```python
from build123d import *

# Parameters (mm, degrees)
F0_W     = 13
F0_H     = 25
F0_W_2   = 20
F0_H_2   = 15
F1_DEPTH = 2


with BuildPart() as f1:
    # F0 (on Front) → F1 (new body)
    with BuildSketch(Plane.XZ):
        Polygon((40.276188, 34.517385), (-59.723812, 34.517385), (-59.723812, -33.482615), (-43.465011, -33.482615), (-43.465011, -10.482615), (-32.465011, -10.482615), (-32.465011, -33.482615), (40.276188, -33.482615), align=None)
        with Locations((-6.950044, -12.5)):
            Rectangle(F0_W, F0_H, mode=Mode.SUBTRACT)
        with Locations((15.719853, -12.5)):
            Rectangle(F0_W, F0_H, mode=Mode.SUBTRACT)
        with Locations((-42.465011, 18.383584)):
            Rectangle(F0_W_2, F0_H_2, mode=Mode.SUBTRACT)
        with Locations((-10.450044, 18.383584)):
            Rectangle(F0_W_2, F0_H_2, mode=Mode.SUBTRACT)
        with Locations((18.867977, 18.383584)):
            Rectangle(F0_W_2, F0_H_2, mode=Mode.SUBTRACT)
    extrude(amount=F1_DEPTH)


solid = f1.part
```
Geometry: final body of the model. Coordinates: model frame, mm. A direction names the side the tool comes from. Coordinates: 2 decimals unless noted, no trailing zeros. Order: outer loops, then holes, each group sorted by start corner. A loop starts at its lowest first (then second) coordinate and runs counter-clockwise, first axis right, second up. Notation, with made-up numbers: M 75.5,51.25 L 102.5,51.25 A9 ccw 102.5,56.25 Z; hole C -20,-1.75 d11. An arc over 180 degrees is marked long. Answer as CSV lines item,"result".
Q1. Section C-C on z = -27.5. Return the cut outline in (x, y).
Answers:
outline,"M -59.72,-2 L -43.47,-2 L -43.47,0 L -59.72,0 Z; M -32.47,-2 L 40.28,-2 L 40.28,0 L -32.47,0 Z"
Q2. Set-up query: faces 1 (the flat face through (-10, -2, 1)), 2 (the flat face through (19, -1, 10.884)), 3 (the flat face through (-38, -1, -10.483)). Return all of +Z, -Z, +X, -X, +Y, -Y with unobstructed straight access to the full face (end or side cutting, diameter ignored); none if empty.
Answers:
face 1,"+Z, -Z, +X, -X, -Y"
face 2,"+Y, -Y"
face 3,"-Z, +Y, -Y"
Q3. First-contact query: P1, Ø8, axis at x = -11.5, z = -21, coming from the -Y side; P2, Ø1, axis at x = -41.5, y = -1, coming from the -Z side. Flat tips, straight axial feed; report the tip coordinate or a pass-through.
Answers:
P1,"stops at y = -2"
P2,"stops at z = -10.48"
Q4. Section B-B on x = -38. Return the cut outline in (y, z).
Answers:
outline,"M -2,-10.48 L 0,-10.48 L 0,10.88 L -2,10.88 Z; M -2,25.88 L 0,25.88 L 0,34.52 L -2,34.52 Z"
Q5. Line query: probe 1 along X at (y, z) = (-0.75, -6.5); probe 2 along Z at (x, y) = (-1.5, -1.35); probe 3 along X at (y, z) = (-0.4, -14). Output: solid intervals per line, ascending. Write a range as [from, to].
Answers:
probe 1,"x = [-59.72, -13.45], [-0.45, 9.22], [22.22, 40.28]"
probe 2,"z = [-33.48, -25], [0, 10.88], [25.88, 34.52]"
probe 3,"x = [-59.72, -43.47], [-32.47, -13.45], [-0.45, 9.22], [22.22, 40.28]"
Q6. Section A-A on z = -2.5. Return the cut outline in (x, y).
Answers:
outline,"M -59.72,-2 L -13.45,-2 L -13.45,0 L -59.72,0 Z; M -0.45,-2 L 9.22,-2 L 9.22,0 L -0.45,0 Z; M 22.22,-2 L 40.28,-2 L 40.28,0 L 22.22,0 Z"
Q7. Draft query along Z for faces 4 (the flat face through (8.868, -1, 18)), 5 (the flat face through (-10, 0, 1)), 6 (the flat face through (3, -1, -33.483)). Return one class per face: pulls with the +Z half, pulls with the -Z half, needs draft (parallel to the pull), parting line crosses it, or undercut.
Answers:
face 4,"undercut"
face 5,"needs draft"
face 6,"pulls with the -Z half"
Q8. Section D-D on y = -1.05. Return the cut outline in (x, z), and give its area (3 significant figures).
Answers:
outline,"M -59.72,-33.48 L -43.47,-33.48 L -43.47,-10.48 L -32.47,-10.48 L -32.47,-33.48 L 40.28,-33.48 L 40.28,34.52 L -59.72,34.52 Z; hole M -52.47,10.88 L -32.47,10.88 L -32.47,25.88 L -52.47,25.88 Z; hole M -20.45,10.88 L -0.45,10.88 L -0.45,25.88 L -20.45,25.88 Z; hole M -13.45,-25 L -0.45,-25 L -0.45,0 L -13.45,0 Z; hole M 8.87,10.88 L 28.87,10.88 L 28.87,25.88 L 8.87,25.88 Z; hole M 9.22,-25 L 22.22,-25 L 22.22,0 L 9.22,0 Z"
area,"5,000 mm^2"
